Work out the finished part from the listing and answer in its coordinate system (mm). Coordinates: 2 decimals unless noted, no trailing zeros. Write each loop counter-clockwise with the first axis right and the second up, starting at its lowest first coordinate (ties: lowest second). Pieces come first, ordered by that corner, then holes. Notation, with made-up numbers: (-24, 55.5) - (-11, 55.5) arc R9 cw to (-11, 59.5) - close; hole circle Ø3 at (37.25, -12.5). An arc over 180 degrees is marked (long way). One line per item, written item: value.
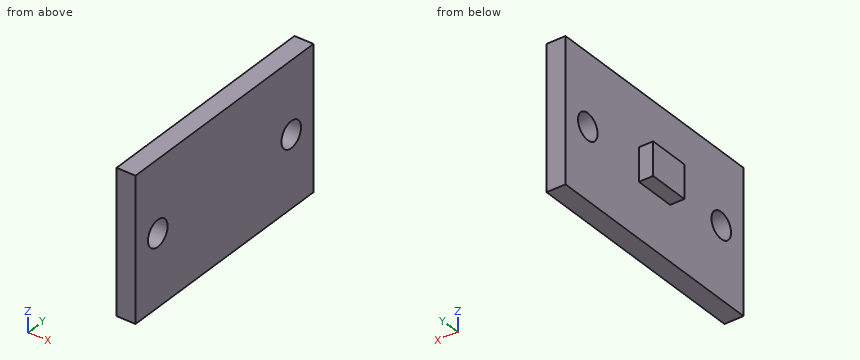
```python
from build123d import *

# Parameters (mm, degrees)
SKETCH1_W           = 12
SKETCH1_H           = 20
BOARD_DEPTH         = 1.6
SKETCH2_W           = 2.8
SKETCH2_H           = 3.5
UV_SENSOR_DEPTH     = 1.2
HOLES_M2_DEPTH      = 12.771151176
HOLES_M2_DEPTH_BACK = 12.771151176
SKETCH3_R           = 1.1


with BuildPart() as part:
    # Sketch1 → Board (new body)
    with BuildSketch(Plane(origin=(0, 0, 0), x_dir=(0, 0, -1), z_dir=(1, 0, 0))):
        Rectangle(SKETCH1_W, SKETCH1_H)
    extrude(amount=BOARD_DEPTH)

    # Sketch2 → UV_Sensor (add)
    with BuildSketch(Plane(origin=(0, 0, 0), x_dir=(0, 0, -1), z_dir=(1, 0, 0))):
        Rectangle(SKETCH2_W, SKETCH2_H)
    extrude(amount=-UV_SENSOR_DEPTH)

    # Sketch3 → Holes_M2 (cut, two sides: drawn at the far end of the back side and taken through both)
    with BuildSketch(Plane(origin=(0, 0, 0), x_dir=(0, 0, -1), z_dir=(1, 0, 0)).offset(-HOLES_M2_DEPTH_BACK)):
        with Locations(Location((0, -7.5, 0), (0, 0, 180))):
            Circle(SKETCH3_R)
        with Locations(Location((0, 7.5, 0), (0, 0, 180))):
            Circle(SKETCH3_R)
    extrude(amount=HOLES_M2_DEPTH + HOLES_M2_DEPTH_BACK, mode=Mode.SUBTRACT)


solid = part.part
```
Item 1: Given pin 1 (0.6 mm diameter, centred on x = -0.5, z = -0.5, fed in from -Y); pin 2 (2.5 mm diameter, centred on y = -7.5, z = 0, fed in from -X), each flat-ended and moving along its own axis, determine where each tip first touches the part or whether it passes through.
Evaluation:
pin 1: stops at y = -1.75
pin 2: stops at x = 0
Item 2: Section C-C, the plane x = 0.2 is taken. Determine the outline of the cut face in (y, z).
Evaluation:
outline: (-10, -6) - (10, -6) - (10, 6) - (-10, 6) - close; hole circle Ø2.2 at (-7.5, 0); hole circle Ø2.2 at (7.5, 0)
Item 3: Consider probe 1 along Y at (x, z) = (0.6, 0); probe 2 along X at (y, z) = (5.5, 2); probe 3 along Z at (x, y) = (-0.2, 0.75). Determine where each line is inside the solid, lowest interval first.
Evaluation:
probe 1: y = -10 to -8.6, -6.4 to 6.4, 8.6 to 10
probe 2: x = 0 to 1.6
probe 3: z = -1.4 to 1.4
Item 4: Section D-D, the plane y = -5 is taken. Determine the outline of the cut face in (x, z), then the cut area to 3 significant figures.
Evaluation:
outline: (0, -6) - (1.6, -6) - (1.6, 6) - (0, 6) - close
area: 19.2 mm2
Item 5: Section B-B, the plane z = 0 is taken. Determine the outline of the cut face in (x, y), then the cut area to 3 significant figures.
Evaluation:
outline: (-1.2, -1.75) - (0, -1.75) - (0, -6.4) - (1.6, -6.4) - (1.6, 6.4) - (0, 6.4) - (0, 1.75) - (-1.2, 1.75) - close; (0, -10) - (1.6, -10) - (1.6, -8.6) - (0, -8.6) - close; (0, 8.6) - (1.6, 8.6) - (1.6, 10) - (0, 10) - close
area: 29.2 mm2
Item 6: Section A-A, the plane y = -7.5 is taken. Determine the outline of the cut face in (x, z).
Evaluation:
outline: (0, -6) - (1.6, -6) - (1.6, -1.1) - (0, -1.1) - close; (0, 1.1) - (1.6, 1.1) - (1.6, 6) - (0, 6) - close
